The model under review builds one solid part; all positions refer to its coordinate system, in mm. Round coordinates to 2 decimals unless told otherwise and drop trailing zeros. Loops run counter-clockwise (first coordinate to the right, second up) from the corner with the lowest first, then second, coordinate; pieces in that order, holes last. Notation, with made-up numbers: (36.5, 69.5) -> (68.5, 69.5) arc R20 ccw to (68.5, 104.5) -> close; hole circle Ø6 at (34, 55). An arc over 180 degrees is marked (long way). Return JSON: item names as keys, results as strings. Group by question number.
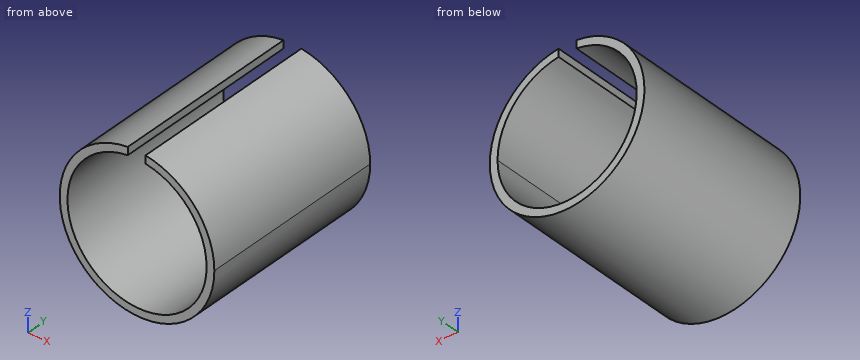
```python
from build123d import *

# Parameters (mm, degrees)
F1_DEPTH = 60


with BuildPart() as f1:
    # F0 (on Front) → F1 (new body)
    with BuildSketch(Plane.XZ):
        with BuildLine():
            ThreePointArc((2.7394399513, 22.3326099853), (16.8506290521, 14.9099396561), (22.5, 0))
            ThreePointArc((22.5, 0), (-14.8113132436, -16.937384686), (-3, 22.299103121))
            Line((-3, 22.299103121), (-3, 24.819347292))
            ThreePointArc((-3, 24.819347292), (-16.5831239518, -18.7082869339), (25, 0))
            ThreePointArc((25, 0), (18.6210364747, 16.6810371563), (2.7394399513, 24.8494561058))
            Line((2.7394399513, 24.8494561058), (2.7394399513, 22.3326099853))
        make_face()
    extrude(amount=F1_DEPTH)


solid = f1.part
```
1. Wall thickness on line 1 (X direction, y = -28, z = -0.5) (3 decimals); line 2 (Z direction, x = 0, y = -30); line 3 (X direction, y = -27, z = -10): over which ranges is each line inside the solid? List them lowest first.
2. We need section B-B, the plane x = -7. Write out the cut boundary in (y, z).
3. We need section A-A, the plane z = 2. Write out the cut boundary in (x, y).
4. We need section C-C, the plane y = -16.5. Write out the cut boundary in (x, z).
5. We need section D-D, the plane x = 0. Write out the cut boundary in (y, z), then the cut area to 3 significant figures.
6. For P1, Ø5, axis at y = -49.5, z = -12, coming from the -X side; P2, Ø3, axis at y = -37, z = 23, coming from the -X side; P3, Ø10, axis at x = 14.5, y = -39.5, coming from the -Z side; P4, Ø8, axis at x = 16, z = 1.5, coming from the +Y side, all flat-tipped, find the tip position at first contact; note any pin that passes through.
Check sheet entries:
{
 "1": {"line 1": "x = -24.995 to -22.494, 22.494 to 24.995", "line 2": "z = -25 to -22.5", "line 3": "x = -22.91 to -20.16, 20.16 to 22.91"},
 "2": {"outline": "(-60, -24) -> (0, -24) -> (0, -21.38) -> (-60, -21.38) -> close; (-60, 21.38) -> (0, 21.38) -> (0, 24) -> (-60, 24) -> close"},
 "3": {"outline": "(-24.92, -60) -> (-22.41, -60) -> (-22.41, 0) -> (-24.92, 0) -> close; (22.41, -60) -> (24.92, -60) -> (24.92, 0) -> (22.41, 0) -> close"},
 "4": {"outline": "(-3, 22.3) -> (-3, 24.82) arc R25 ccw (long way) to (2.74, 24.85) -> (2.74, 22.33) arc R22.5 cw (long way) to start"},
 "5": {"outline": "(-60, -25) -> (0, -25) -> (0, -22.5) -> (-60, -22.5) -> close", "area": "150 mm²"},
 "6": {"P1": "stops at x = -23.12", "P2": "stops at x = -12.76", "P3": "stops at z = -23.12", "P4": "passes through"}
}
